Geometry check sheet. Reference: the model listing, model coordinates, mm. Give positions to 0.01 mm unless a question says otherwise; leave off trailing zeros. Loops run counter-clockwise (first coordinate to the right, second up) from the corner with the lowest first, then second, coordinate; pieces in that order, holes last. Notation, with made-up numbers: (12.5, 2) -> (34.5, 2) arc R32 cw to (34.5, 38) -> close; hole circle Ø5 at (73, 51). An arc over 180 degrees is marked (long way). One line per question, with ' | ' between items.
from build123d import *

# Parameters (mm, degrees)
SKETCH1_W           = 12
SKETCH1_H           = 100
SKETCH1_R           = 2
BOSS_EXTRUDE1_DEPTH = 5


with BuildPart() as part:
    # Sketch1 → Boss-Extrude1 (new body)
    with BuildSketch(Plane.XY):
        Rectangle(SKETCH1_W, SKETCH1_H)
        Circle(SKETCH1_R, mode=Mode.SUBTRACT)
        with Locations((0, 10)):
            Circle(SKETCH1_R, mode=Mode.SUBTRACT)
        with Locations((0, 20)):
            Circle(SKETCH1_R, mode=Mode.SUBTRACT)
        with Locations((0, 30)):
            Circle(SKETCH1_R, mode=Mode.SUBTRACT)
        with Locations((0, 40)):
            Circle(SKETCH1_R, mode=Mode.SUBTRACT)
        with Locations((0, -10)):
            Circle(SKETCH1_R, mode=Mode.SUBTRACT)
        with Locations((0, -20)):
            Circle(SKETCH1_R, mode=Mode.SUBTRACT)
        with Locations((0, -30)):
            Circle(SKETCH1_R, mode=Mode.SUBTRACT)
        with Locations((0, -40)):
            Circle(SKETCH1_R, mode=Mode.SUBTRACT)
    extrude(amount=BOSS_EXTRUDE1_DEPTH)


solid = part.part
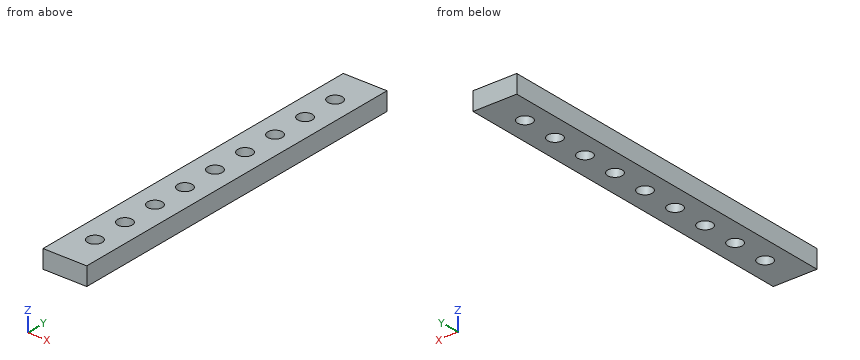
Item 1: Sectioned sample at B-B (z = 3.6). Give the number of separate pieces and of enclosed holes in the cut face, plus the area to 3 significant figures.
Result:
separate pieces: 1 | enclosed holes: 9 | area: 1,090 mm2
Item 2: Scan line: probe 1 along X at (y, z) = (-41, 3.65). Record every from-to range of solid material in increasing order.
Result:
probe 1: -6 to -1.73, 1.73 to 6
Item 3: Sectioned sample at A-A (y = -10). Record the cut outline in (x, z), plus the area to 3 significant figures.
Result:
outline: (-6, 0) -> (-2, 0) -> (-2, 5) -> (-6, 5) -> close; (2, 0) -> (6, 0) -> (6, 5) -> (2, 5) -> close | area: 40.0 mm2
